Print and shaded views of the part. All mm, measured from the part's lowest x, y and z. Round coordinates to 2 decimals unless told otherwise and drop trailing zeros. Write each loop counter-clockwise with the first axis right and the second up, starting at its lowest first coordinate (ties: lowest second). Pieces come first, ordered by that corner, then holes. Notation, with made-up numbers: (43, 56) - (47, 56) arc R22 cw to (47, 73) - close; hole circle Ø8 at (-11, -32.75). An arc over 180 degrees is marked (long way). One line per item, written item: value.
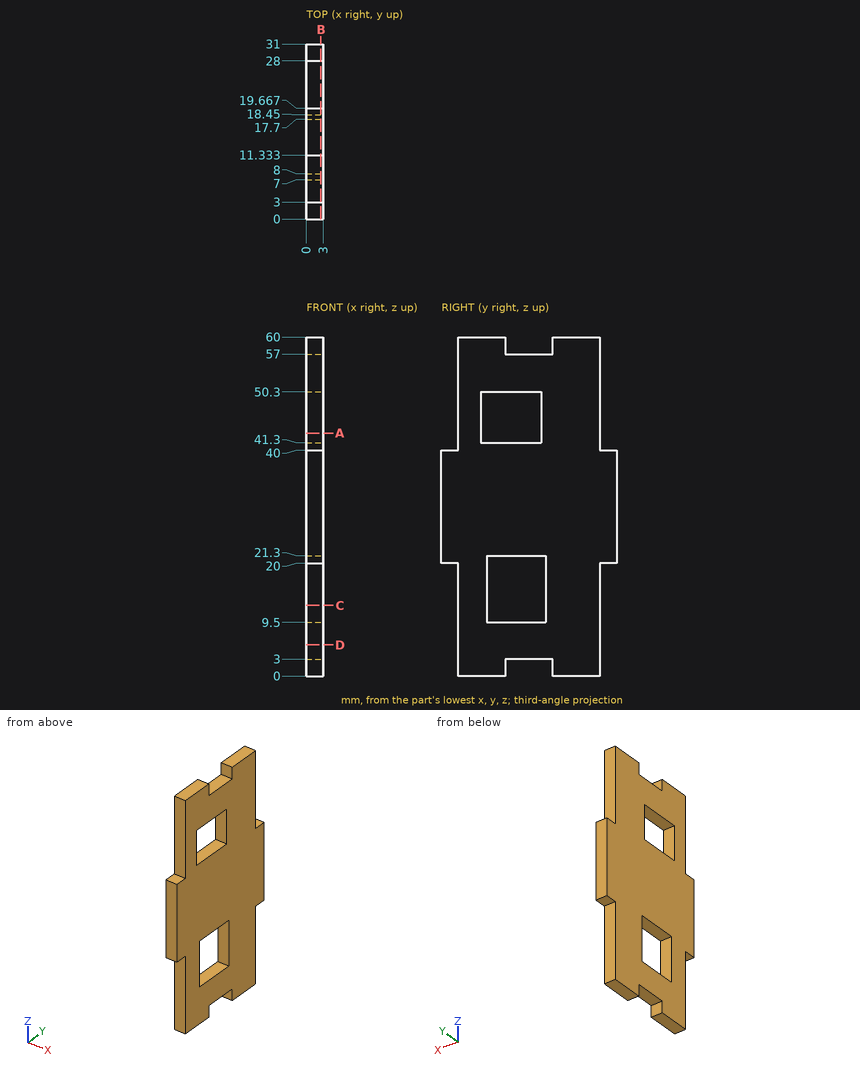
1. Band-saw the part on A-A on z = 43. Write the cut outline in (x, y).
Report:
outline: (0, 3) - (3, 3) - (3, 7) - (0, 7) - close; (0, 17.7) - (3, 17.7) - (3, 28) - (0, 28) - close
2. Band-saw the part on C-C on z = 12.5. Write the cut outline in (x, y).
Report:
outline: (0, 3) - (3, 3) - (3, 8) - (0, 8) - close; (0, 18.45) - (3, 18.45) - (3, 28) - (0, 28) - close
3. Wall check: probe 1 along Z at (x, y) = (1.75, 11.5); probe 2 along Y at (x, z) = (2.6, 43); probe 3 along Y at (x, z) = (1.25, 18). Give the ranges that are in metal, low to high. Write a range as [from, to].
Report:
probe 1: [3, 9.5], [21.3, 41.3], [50.3, 57]
probe 2: [3, 7], [17.7, 28]
probe 3: [3, 8], [18.45, 28]
4. Band-saw the part on D-D on z = 5.5. Write the cut outline in (x, y).
Report:
outline: (0, 3) - (3, 3) - (3, 28) - (0, 28) - close
5. Drop flat-ended pins along their axis: pin 1 (1.5 mm diameter, centred on x = 1.5, z = 46.5, fed in from +Y); pin 2 (0.9 mm diameter, centred on x = 2, y = 1.5, fed in from +Z); pin 3 (1.5 mm diameter, centred on x = 1, y = 14.5, fed in from -Z). Give the stop position or say it passes through.
Report:
pin 1: y = 28
pin 2: z = 40
pin 3: z = 3
6. Band-saw the part on B-B on x = 2.55. Write the cut outline in (y, z).
Report:
outline: (0, 20) - (3, 20) - (3, 0) - (11.33, 0) - (11.33, 3) - (19.67, 3) - (19.67, 0) - (28, 0) - (28, 20) - (31, 20) - (31, 40) - (28, 40) - (28, 60) - (19.67, 60) - (19.67, 57) - (11.33, 57) - (11.33, 60) - (3, 60) - (3, 40) - (0, 40) - close; hole (7, 41.3) - (17.7, 41.3) - (17.7, 50.3) - (7, 50.3) - close; hole (8, 9.5) - (18.45, 9.5) - (18.45, 21.3) - (8, 21.3) - close
